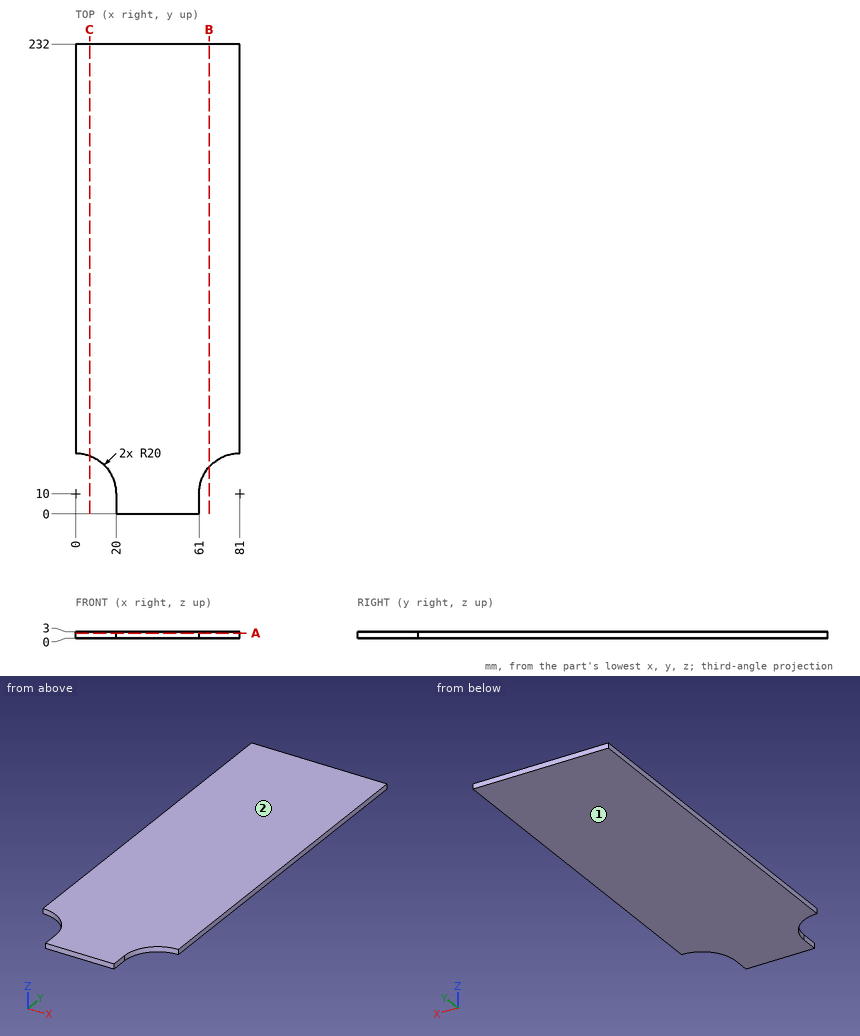
Can you work these out from the drawing? Everything is in mm from the part's minimum corner. Round coordinates to 2 decimals unless told otherwise and drop trailing zeros. Write each loop counter-clockwise with the first axis right and the second up, starting at its lowest first coordinate (ties: lowest second). Pieces come first, ordered by that corner, then holes.
1. If we mould it in two halves opening along Z, with no side actions, what happens to the marked faces 1 and 2? For each: released by +Z, released by -Z, zero draft, split by the parting line, or undercut.
2. Suppose I cut it at C-C (x = 7). List the corners of the cut face in (y, z) for me (3 decimals).
3. Suppose I cut it at A-A (z = 2.4). List the corners of the cut face in (x, y) for me, and give its area (3 significant figures).
4. Will this pin go through, and if not, where does the flat tip stop? pin 1 Ø0.9 at (y, z) = (7, 2) entering from -X.
5. I need wall thicknesses on L1, parallel to Y at x = 64.5, z = 0.85; L2, parallel to Y at x = 5, z = 2.7. Which ranges of each line are inside material? Lowest first, please.
6. Suppose I cut it at B-B (x = 66). List the corners of the cut face in (y, z) for me.
Answer sheet:
1. face 1: released by -Z
1. face 2: released by +Z
2. outline: (28.735, 0) - (232, 0) - (232, 3) - (28.735, 3) - close
3. outline: (0, 30) arc R20 cw to (20, 10) - (20, 0) - (61, 0) - (61, 10) arc R20 cw to (81, 30) - (81, 232) - (0, 232) - close
3. area: 17,800 mm2
4. pin 1: stops at x = 20
5. L1: y = 21.3 to 232
5. L2: y = 29.36 to 232
6. outline: (23.23, 0) - (232, 0) - (232, 3) - (23.23, 3) - close
